Model file for the job. Use its own axes, mm. A direction names the side the tool comes from. Coordinates: 2 decimals unless noted, no trailing zeros. Loops run counter-clockwise (first coordinate to the right, second up) from the corner with the lowest first, then second, coordinate; pieces in that order, holes last. Notation, with made-up numbers: (83, 24.25) -> (130, 24.25) arc R5 cw to (130, 30.25) -> close; hole circle Ø7 at (81.5, -30.75). An arc over 180 degrees is marked (long way). Use one line per item in the form item = value.
```python
from build123d import *

# Parameters (mm, degrees)
SKETCH_1_R          = 2.5
EXTRUDE_1_DEPTH     = 10
SKETCH_2_R          = 1.5
CUT_EXTRUDE_1_DEPTH = 35.936549629


with BuildPart() as part:
    # Sketch 1 → Extrude 1 (new body)
    with BuildSketch(Plane.XY):
        with BuildLine():
            ThreePointArc((17.185510359, 7.497413467), (21.249009569, 2.10671914), (17.388376345, -3.431071237))
            Line((17.388376345, -3.431071237), (10, -6))
            Line((10, -6), (10, -12))
            Line((10, -12), (0.5, -12))
            Line((0.5, -12), (0.5, -6))
            Line((0.5, -6), (0.5, -1.968626967))
            ThreePointArc((0.5, -1.968626967), (0, 6), (-0.5, -1.968626967))
            Line((-0.5, -1.968626967), (-0.5, -6))
            Line((-0.5, -6), (-0.5, -12))
            Line((-0.5, -12), (-10, -12))
            Line((-10, -12), (-10, -6))
            Line((-10, -6), (-17.388376345, -3.431071237))
            ThreePointArc((-17.388376345, -3.431071237), (-21.249009569, 2.10671914), (-17.185510359, 7.497413467))
            Line((-17.185510359, 7.497413467), (-2.5, 12))
            Line((-2.5, 12), (2.5, 12))
            Line((2.5, 12), (17.185510359, 7.497413467))
        make_face()
        with Locations((-15.5, 2)):
            Circle(SKETCH_1_R, mode=Mode.SUBTRACT)
        with Locations((15.5, 2)):
            Circle(SKETCH_1_R, mode=Mode.SUBTRACT)
    extrude(amount=EXTRUDE_1_DEPTH)

    # Sketch 2 → Cut-Extrude 1 (cut, through all)
    with BuildSketch(Plane(origin=(10, 0, 0), x_dir=(0, 0, -1), z_dir=(1, 0, 0))):
        with Locations(Location((-5, -9, 0), (0, 0, 90))):
            Circle(SKETCH_2_R)
    extrude(amount=-CUT_EXTRUDE_1_DEPTH, mode=Mode.SUBTRACT)


solid = part.part
```
Q1. Wall check: line 1 along X through (y, z) = (4, 9.25); line 2 along X through (y, z) = (0.75, 5.25); line 3 along Y through (x, z) = (0, 5.5). Give the ranges that are in metal, low to high.
Result:
line_1 = -20.89 to -17, -14 to -3.46, 3.46 to 14, 17 to 20.89
line_2 = -21.11 to -17.67, -13.33 to -3.8, 3.8 to 13.33, 17.67 to 21.11
line_3 = 6 to 12
Q2. Band-saw the part on D-D, the plane x = -15.5. Write the cut outline in (y, z), and give its area (3 significant figures).
Result:
outline = (-4.09, 0) -> (-0.5, 0) -> (-0.5, 10) -> (-4.09, 10) -> close; (4.5, 0) -> (8.01, 0) -> (8.01, 10) -> (4.5, 10) -> close
area = 71.0 mm2
Q3. Band-saw the part on C-C, the plane y = -1.25. Write the cut outline in (x, z).
Result:
outline = (-20.24, 0) -> (-2.33, 0) -> (-2.33, 10) -> (-20.24, 10) -> close; (2.33, 0) -> (20.24, 0) -> (20.24, 10) -> (2.33, 10) -> close
Q4. Mould opens along Y. For faces 4 (the face through (10, -10.3, 3.8)), 5 (the face through (-5.18, -10.5, 5.07)), 6 (the face through (-5, -12, 5)), 7 (the face through (-18, 2, 5)) say: released by +Y, released by -Y, zero draft, split by the parting line, or undercut.
Result:
face_4 = zero draft
face_5 = undercut
face_6 = released by -Y
face_7 = undercut
Q5. Band-saw the part on B-B, the plane z = 4. Write the cut outline in (x, y).
Result:
outline = (-17.39, -3.43) -> (-10, -6) -> (-10, -7.88) -> (-0.5, -7.88) -> (-0.5, -1.97) arc R4 cw (long way) to (0.5, -1.97) -> (0.5, -7.88) -> (10, -7.88) -> (10, -6) -> (17.39, -3.43) arc R5.75 ccw to (17.19, 7.5) -> (2.5, 12) -> (-2.5, 12) -> (-17.19, 7.5) arc R5.75 ccw to start; (-10, -12) -> (-0.5, -12) -> (-0.5, -10.12) -> (-10, -10.12) -> close; (0.5, -12) -> (10, -12) -> (10, -10.12) -> (0.5, -10.12) -> close; hole circle Ø5 at (-15.5, 2); hole circle Ø5 at (15.5, 2)
Q6. Which spindle directions (+Z, -Z, +X, -X, +Y, -Y) get a long thin tool onto all of the face, cutting with end or side? Do faces 1 (the face through (-10, -7.7, 3.8)), 2 (the face through (5.32, -10.5, 5.07)), 3 (the face through (-0.5, -7, 5)). Say none if no direction does.
Result:
face_1 = +Z, -Z, -X, -Y
face_2 = +X, -X
face_3 = +Z, -Z, -Y
Q7. Band-saw the part on A-A, the plane y = -9. Write the cut outline in (x, z), and give its area (3 significant figures).
Result:
outline = (-10, 0) -> (-0.5, 0) -> (-0.5, 3.5) -> (-10, 3.5) -> close; (-10, 6.5) -> (-0.5, 6.5) -> (-0.5, 10) -> (-10, 10) -> close; (0.5, 0) -> (10, 0) -> (10, 3.5) -> (0.5, 3.5) -> close; (0.5, 6.5) -> (10, 6.5) -> (10, 10) -> (0.5, 10) -> close
area = 133 mm2
Q8. Pin check, flat tips, straight feed: pin 1 Ø4 at (y, z) = (-9, 5) entering from -X; pin 2 Ø1.8 at (y, z) = (-10, 3.5) entering from +X; pin 3 Ø5 at (x, z) = (14, 3.5) entering from +Y. Stop position of each tip, or through.
Result:
pin_1 = -10
pin_2 = 10
pin_3 = 9.24
